Check sheet for the modelled part. Datum: model origin and axes. Units: mm. A direction names the side the tool comes from. Round coordinates to 2 decimals unless told otherwise and drop trailing zeros. Write each loop counter-clockwise with the first axis right and the second up, starting at its lowest first coordinate (ties: lowest second). Pieces come first, ordered by that corner, then holes.
Item 1: Material ranges on line 1 along X through (y, z) = (0.5, 19); line 2 along Z through (x, y) = (36.5, 1.25); line 3 along Y through (x, z) = (49.5, 13.25), recorded low to high.
Item 2: Set-up check for faces 1 (the flat face through (6, -4.5, 12)), 2 (the cylindrical face through (65.705, -2.218, 12.727)), 3 (the cylindrical face through (36.764, 1.479, 7.235)): record each of +Z, -Z, +X, -X, +Y, -Y from which the full face is reachable in a straight line by a thin tool's end or side.
Item 3: Section check C-C, the plane z = 18. Record the cut outline in (x, y).
Item 4: Depth check by flat-ended pin: pin 1 (4 mm diameter, centred on x = 57.5, z = 11, fed in from -Y); pin 2 (2 mm diameter, centred on y = -2.5, z = 17.5, fed in from +X); pin 3 (4 mm diameter, centred on y = 1, z = 15.5, fed in from +X); pin 4 (1.5 mm diameter, centred on y = 1, z = 14, fed in from -X). Enter the tip coordinate at first touch or a pass-through.
Item 5: Section check A-A, the plane z = 12. Record the cut outline in (x, y), plus the area to 3 significant figures.
Item 6: Section check D-D, the plane x = 7. Record the cut outline in (y, z).
Item 7: Section check B-B, the plane y = 1.5. Record the cut outline in (x, z), plus the area to 3 significant figures.
Item 8: Release check for a two-part mould opening along Z. For faces 4 (the cylindrical face through (68.99, -0.61, 12.97)), 5 (the flat face through (53.1, 1.48, 17.39)), 6 (the flat face through (36, 3, 7)), 7 (the flat face through (38.399, 1, 14)) record: pulls with the +Z half, pulls with the -Z half, needs draft (parallel to the pull), parting line crosses it, or undercut.
from build123d import *

# Parameters (mm, degrees)
BOSS_EXTRUDE1_DEPTH = 3
SKETCH1_3_R         = 1.8
BOSS_EXTRUDE2_DEPTH = 4.5
BOSS_EXTRUDE3_START = -1.2
SKETCH1_4_R         = 3.998679456
SKETCH1_4_R_2       = 2
SKETCH1_4_R_3       = 4.002518736
BOSS_EXTRUDE3_DEPTH = 1.2


with BuildPart() as part:
    # Sketch1 → Boss-Extrude1 (new body)
    with BuildSketch(Plane(origin=(0, 0, 0), x_dir=(1, 0, 0), z_dir=(0, 1, 0))):
        with BuildLine():
            Line((6.299371737, -15.895179228), (34.299371737, -18.834953384))
            ThreePointArc((34.299371737, -18.834953384), (36.799371737, -21.334953384), (39.299371737, -18.834953384))
            Line((39.299371737, -18.834953384), (67.302380501, -15.899018508))
            ThreePointArc((67.302380501, -15.899018508), (71.304899237, -11.896499772), (67.302380501, -7.893981036))
            Line((67.302380501, -7.893981036), (36.799371737, -6.334953384))
            Line((36.799371737, -6.334953384), (6.299371737, -7.897820316))
            ThreePointArc((6.299371737, -7.897820316), (2.300692281, -11.896499772), (6.299371737, -15.895179228))
        make_face()
        with BuildLine():
            ThreePointArc((35.199371737, -8.834953384), (36.799371737, -7.234953384), (38.399371737, -8.834953384))
            Line((38.399371737, -8.834953384), (38.399371737, -18.834953384))
            ThreePointArc((38.399371737, -18.834953384), (36.799371737, -20.434953384), (35.199371737, -18.834953384))
            Line((35.199371737, -18.834953384), (35.199371737, -8.834953384))
        make_face(mode=Mode.SUBTRACT)
    extrude(amount=BOSS_EXTRUDE1_DEPTH)

    # Sketch1_3 → Boss-Extrude2 (add)
    with BuildSketch(Plane(origin=(0, 0, 0), x_dir=(1, 0, 0), z_dir=(0, 1, 0))):
        with Locations(Location((6.299371737, -11.896499772, 0), (0, 0, 270))):
            Circle(SKETCH1_3_R)
        with Locations(Location((67.302380501, -11.896499772, 0), (0, 0, 270))):
            Circle(SKETCH1_3_R)
    extrude(amount=-BOSS_EXTRUDE2_DEPTH)

    # Sketch1_4 → Boss-Extrude3 (add)
    # profile 1 of 2: a face of its own
    with BuildSketch(Plane(origin=(0, 0, 0), x_dir=(1, 0, 0), z_dir=(0, 1, 0)).offset(BOSS_EXTRUDE3_START)):
        with Locations(Location((6.299371737, -11.896499772, 0), (0, 0, 270))):
            Circle(SKETCH1_4_R)
        with Locations(Location((6.299371737, -11.896499772, 0), (0, 0, 270))):
            Circle(SKETCH1_4_R_2, mode=Mode.SUBTRACT)
    # profile 2 of 2: a face of its own
    with BuildSketch(Plane(origin=(0, 0, 0), x_dir=(1, 0, 0), z_dir=(0, 1, 0)).offset(BOSS_EXTRUDE3_START)):
        with Locations(Location((67.302380501, -11.896499772, 0), (0, 0, 270))):
            Circle(SKETCH1_4_R_3)
        with Locations(Location((67.302380501, -11.896499772, 0), (0, 0, 270))):
            Circle(SKETCH1_4_R_2, mode=Mode.SUBTRACT)
    extrude(amount=BOSS_EXTRUDE3_DEPTH)


solid = part.part
Values found:
1. line 1: x = 34.3 to 35.21, 38.39 to 39.29
1. line 2: z = 6.35 to 7.26, 20.41 to 21.32
1. line 3: y = 0 to 3
2. face 1: +Z, -Z, +X, -X, -Y
2. face 2: -Y
2. face 3: +Y, -Y
3. outline: (26.35, 0) - (35.2, 0) - (35.2, 3) - (26.35, 3) - close; (38.4, 0) - (47.26, 0) - (47.26, 3) - (38.4, 3) - close
4. pin 1: stops at y = 0
4. pin 2: passes through
4. pin 3: stops at x = 70.97
4. pin 4: stops at x = 2.54
5. outline: (2.3, -1.2) - (4.3, -1.2) - (4.3, 0) - (4.5, 0) - (4.5, -4.5) - (8.1, -4.5) - (8.1, 0) - (8.3, 0) - (8.3, -1.2) - (10.3, -1.2) - (10.3, 0) - (35.2, 0) - (35.2, 3) - (2.3, 3) - close; (38.4, 0) - (63.3, 0) - (63.3, -1.2) - (65.31, -1.2) - (65.31, 0) - (65.51, 0) - (65.51, -4.5) - (69.1, -4.5) - (69.1, 0) - (69.3, 0) - (69.3, -1.2) - (71.3, -1.2) - (71.3, 3) - (38.4, 3) - close
5. area: 239 mm2
6. outline: (-4.5, 10.24) - (0, 10.24) - (0, 10.02) - (-1.2, 10.02) - (-1.2, 7.96) - (0, 7.96) - (0, 7.86) - (3, 7.86) - (3, 15.97) - (0, 15.97) - (0, 15.83) - (-1.2, 15.83) - (-1.2, 13.77) - (0, 13.77) - (0, 13.55) - (-4.5, 13.55) - close
7. outline: (6.3, 7.9) - (36.8, 6.33) - (67.3, 7.89) arc R4 ccw to (67.3, 15.9) - (39.3, 18.83) arc R2.5 ccw to (34.3, 18.83) - (6.3, 15.9) arc R4 ccw to start; hole (35.2, 8.83) arc R1.6 ccw to (38.4, 8.83) - (38.4, 18.83) arc R1.6 ccw to (35.2, 18.83) - close
7. area: 653 mm2
8. face 4: undercut
8. face 5: pulls with the +Z half
8. face 6: needs draft
8. face 7: undercut
